Geometry: final body of the model. Coordinates: model frame, mm. A direction names the side the tool comes from. Coordinates: 2 decimals unless noted, no trailing zeros. Order: outer loops, then holes, each group sorted by start corner. A loop starts at its lowest first (then second) coordinate and runs counter-clockwise, first axis right, second up. Notation, with made-up numbers: (52, -25) - (111, -25) arc R13 ccw to (111, -4) - close; hole circle Ø8 at (15, 59.25). An arc over 180 degrees is marked (long way). Use a Markdown table: item, result. Add a question column.
```python
from build123d import *

# Parameters (mm, degrees)
SKETCH022_W            = 64
SKETCH022_H            = 64
PAD020_DEPTH           = 9
SKETCH023_R            = 1.6
POCKET003_DEPTH        = 9
SKETCH024_R            = 1.6
POCKET004_DEPTH        = 9
SKETCH025_R            = 3
POCKET005_DEPTH        = 5.5
SKETCH026_R            = 4.5
POCKET006_DEPTH        = 9
SKETCH030_R            = 1.55
POCKET009_DEPTH        = 9
SKETCH031_W            = 30
SKETCH031_H            = 27.227398
PAD022_DEPTH           = 9
SKETCH032_R            = 1.55
POCKET010_DEPTH        = 9
SKETCH066_W            = 16.8
SKETCH066_H            = 9
PAD040_DEPTH           = 8
PAD040_FACE8_W         = 9
PAD040_FACE8_H         = 16
PAD041_DEPTH           = 7
MIRRORED_FACE11_W      = 9
MIRRORED_FACE11_H      = 18
PAD042_DEPTH           = 7
PAD043_DEPTH           = 5.8
SKETCH068_R            = 2
POCKET027_DEPTH        = 5
LINEARPATTERN_COUNT    = 3
LINEARPATTERN_PITCH    = 6.4
SKETCH069_R            = 2
POCKET028_DEPTH        = 5
LINEARPATTERN001_COUNT = 3
LINEARPATTERN001_PITCH = 6.4
SKETCH071_W            = 10
SKETCH071_H            = 4
PAD044_DEPTH           = 5.8
SKETCH073_R            = 2
POCKET029_DEPTH        = 100
SKETCH074_W            = 11
SKETCH074_H            = 6
PAD045_DEPTH           = 50
SKETCH075_W            = 11
SKETCH075_H            = 2
POCKET030_DEPTH        = 12
SKETCH076_R            = 1.6
POCKET031_DEPTH        = 10
SKETCH083_R            = 3.25
POCKET035_DEPTH        = 4


with BuildPart() as part:
    # Sketch022 → Pad020 (new body)
    with BuildSketch(Plane.XZ):
        Rectangle(SKETCH022_W, SKETCH022_H)
    extrude(amount=PAD020_DEPTH)

    # Sketch023 (on Face5 of Pad020) → Pocket003 (cut)
    with BuildSketch(Plane(origin=(0, 0, 0), x_dir=(1, 0, 0), z_dir=(0, 1, 0))):
        with Locations((-9.5, 7.5)):
            Circle(SKETCH023_R)
        with Locations((-23.5, 7.5)):
            Circle(SKETCH023_R)
    extrude(amount=-POCKET003_DEPTH, mode=Mode.SUBTRACT)

    # Sketch024 (on Face4 of Pocket003) → Pocket004 (cut)
    with BuildSketch(Plane(origin=(0, 0, 0), x_dir=(1, 0, 0), z_dir=(0, 1, 0))):
        with Locations((1.4, 17.5)):
            Circle(SKETCH024_R)
        with Locations((18.9, -1.5)):
            Circle(SKETCH024_R)
    extrude(amount=-POCKET004_DEPTH, mode=Mode.SUBTRACT)

    # Sketch025 (on Face4 of Pocket004) → Pocket005 (cut)
    with BuildSketch(Plane(origin=(0, 0, 0), x_dir=(1, 0, 0), z_dir=(0, 1, 0))):
        with Locations((-23.5, 7.5)):
            Circle(SKETCH025_R)
        with Locations((-9.5, 7.5)):
            Circle(SKETCH025_R)
    extrude(amount=-POCKET005_DEPTH, mode=Mode.SUBTRACT)

    # Sketch026 (on Face4 of Pocket005) → Pocket006 (cut)
    with BuildSketch(Plane(origin=(0, 0, 0), x_dir=(1, 0, 0), z_dir=(0, 1, 0))):
        with Locations((0, -20)):
            Circle(SKETCH026_R)
        with Locations((20, 20)):
            Circle(SKETCH026_R)
        with Locations((-20, 20)):
            Circle(SKETCH026_R)
    extrude(amount=-POCKET006_DEPTH, mode=Mode.SUBTRACT)

    # Sketch030 (on Face5 of Pocket006) → Pocket009 (cut)
    with BuildSketch(Plane.XZ.offset(9)):
        with Locations((7.5, -7.5)):
            Circle(SKETCH030_R)
    extrude(amount=-POCKET009_DEPTH, mode=Mode.SUBTRACT)

    # Sketch031 (on Face5 of Pocket009) → Pad022 (join)
    with BuildSketch(Plane.XZ.offset(9)):
        with Locations((-1, 45.613699)):
            Rectangle(SKETCH031_W, SKETCH031_H)
    extrude(amount=-PAD022_DEPTH)

    # Sketch032 (on Face22 of Pad022) → Pocket010 (cut)
    with BuildSketch(Plane.XZ.offset(9)):
        with Locations((-9.5, 47.5)):
            Circle(SKETCH032_R)
        with Locations((7.5, 47.5)):
            Circle(SKETCH032_R)
    extrude(amount=-POCKET010_DEPTH, mode=Mode.SUBTRACT)

    # Sketch066 (on Face2 of Pocket010) → Pad040 (join)
    with BuildSketch(Plane(origin=(-32, 0, 0), x_dir=(0, 0, -1), z_dir=(-1, 0, 0))):
        with Locations((-30.6, 4.5)):
            Rectangle(SKETCH066_W, SKETCH066_H)
    pad040 = extrude(amount=PAD040_DEPTH)

    # Pad040 Face8 → Pad041 (add)
    with BuildSketch(Plane(origin=(-24, -4.5, 32), x_dir=(0, 1, 0), z_dir=(0, 0, 1))):
        Rectangle(PAD040_FACE8_W, PAD040_FACE8_H)
    extrude(amount=PAD041_DEPTH)

    # Mirrored: Pad040 across YZ
    add(pad040.mirror(Plane.YZ))

    # Mirrored Face11 → Pad042 (add)
    with BuildSketch(Plane(origin=(23, -4.5, 32), x_dir=(0, 1, 0), z_dir=(0, 0, 1))):
        Rectangle(MIRRORED_FACE11_W, MIRRORED_FACE11_H)
    extrude(amount=PAD042_DEPTH)

    # Sketch067 (on Face27 of Pad042) → Pad043 (join)
    with BuildSketch(Plane.XZ.offset(9)):
        Polygon((40, 39), (32, 39), (32, 22.2), (40, 22.2), (40, 24.2), (34, 24.2), (34, 37), (40, 37), align=None)
    pad043 = extrude(amount=PAD043_DEPTH)

    # Mirrored001: Pad043 across YZ
    add(pad043.mirror(Plane.YZ))

    # Sketch068 (on Face37 of Mirrored001) → Pocket027 (cut)
    with BuildSketch(Plane(origin=(-34, 0, 0), x_dir=(0, 0, -1), z_dir=(-1, 0, 0))):
        with Locations((-24.2, 11.9)):
            Circle(SKETCH068_R)
    pocket027 = extrude(amount=-POCKET027_DEPTH, mode=Mode.SUBTRACT)

    # LinearPattern: Pocket027 ×3
    with Locations(*[(0, 0, i * LINEARPATTERN_PITCH) for i in range(1, LINEARPATTERN_COUNT)]):
        add(pocket027, mode=Mode.SUBTRACT)

    # Sketch069 (on Face44 of LinearPattern) → Pocket028 (cut)
    with BuildSketch(Plane(origin=(34, 0, 0), x_dir=(0, 0, 1), z_dir=(1, 0, 0))):
        with Locations((37, 11.9)):
            Circle(SKETCH069_R)
    pocket028 = extrude(amount=-POCKET028_DEPTH, mode=Mode.SUBTRACT)

    # LinearPattern001: Pocket028 ×3
    with Locations(*[(0, 0, -i * LINEARPATTERN001_PITCH) for i in range(1, LINEARPATTERN001_COUNT)]):
        add(pocket028, mode=Mode.SUBTRACT)

    # Sketch071 (on Face35 of LinearPattern001) → Pad044 (join)
    with BuildSketch(Plane.XZ.offset(9)):
        with Locations((25, 21.7)):
            Rectangle(SKETCH071_W, SKETCH071_H)
        with Locations((25, -28.3)):
            Rectangle(SKETCH071_W, SKETCH071_H)
    pad044 = extrude(amount=PAD044_DEPTH)

    # Mirrored003: Pad044 across Sketch071 V_Axis
    add(pad044.mirror(Plane(origin=(0, -9, 0), x_dir=(0, -1, 0), z_dir=(1, 0, 0))))

    # Sketch073 (on Face49 of Mirrored003) → Pocket029 (cut)
    with BuildSketch(Plane(origin=(0, 0, 23.7), x_dir=(-1, 0, 0), z_dir=(0, 0, 1))):
        with Locations((-25, 11.9)):
            Circle(SKETCH073_R)
    pocket029 = extrude(amount=-POCKET029_DEPTH, mode=Mode.SUBTRACT)

    # Mirrored004: Pocket029 across YZ
    add(pocket029.mirror(Plane.YZ), mode=Mode.SUBTRACT)

    # Sketch074 (on Face15 of Mirrored004) → Pad045 (join)
    with BuildSketch(Plane(origin=(0, 0, -32), x_dir=(1, 0, 0), z_dir=(0, 0, -1))):
        with Locations((0, 3)):
            Rectangle(SKETCH074_W, SKETCH074_H)
    extrude(amount=PAD045_DEPTH)

    # Sketch075 (on Face41 of Pad045) → Pocket030 (cut)
    with BuildSketch(Plane(origin=(5.5, 0, 0), x_dir=(0, 0, 1), z_dir=(1, 0, 0))):
        with Locations((-74.5, 3)):
            Rectangle(SKETCH075_W, SKETCH075_H)
        with Locations((-45.5, 3)):
            Rectangle(SKETCH075_W, SKETCH075_H)
    extrude(amount=-POCKET030_DEPTH, mode=Mode.SUBTRACT)

    # Sketch076 (on Face30 of Pocket030) → Pocket031 (cut)
    with BuildSketch(Plane.XZ.offset(9)):
        with Locations((29, -12.3)):
            Circle(SKETCH076_R)
        with Locations((29, -20.3)):
            Circle(SKETCH076_R)
    extrude(amount=-POCKET031_DEPTH, mode=Mode.SUBTRACT)

    # Sketch083 (on Face32 of Pocket031) → Pocket035 (cut)
    with BuildSketch(Plane.XZ.offset(9)):
        with Locations((1.4, -17.5)):
            Circle(SKETCH083_R)
    extrude(amount=-POCKET035_DEPTH, mode=Mode.SUBTRACT)


solid = part.part
```
1) Line query: line 1 (X direction, y = -11.9, z = 21.95); line 2 (Z direction, x = 7.5, y = -7); line 3 (Y direction, x = -25, z = -27). Output: solid intervals per line, ascending. Write a range as from..to.
2) Draft query along Y for faces 1 (the flat face through (0, -4, -75)), 2 (the flat face through (-22, -5.5, -6)), 3 (the cylindrical face through (3.15, -7.03, -14.76)), 4 (the flat face through (25, -14.8, -28)). Return one class per face: released by +Y, released by -Y, zero draft, split by the parting line, or undercut.
3) Section query C-C (x = 1.4). Return the cut outline in (y, z).
4) First-contact query: pin 1 (7 mm diameter, centred on y = -6, z = 7, fed in from +X); pin 2 (7.5 mm diameter, centred on x = -23, y = -6, fed in from +Z); pin 3 (5.5 mm diameter, centred on x = 2, z = -46.5, fed in from -Y); pin 4 (5.5 mm diameter, centred on x = -2, z = -72.5, fed in from +Y). Flat tips, straight axial feed; report the tip coordinate or a pass-through.
5) Section query B-B (y = -7.5). Give the number of separate pieces and of enclosed holes in the cut face, and give its area (3 significant figures).
6) Section query A-A (z = -7.5). Return the cut outline in (x, y).
7) Access query for faces 5 (the flat face through (37, -12, 24.2)), 6 (the cylindrical face through (33.014, -9.948, 36.566)), 7 (the flat face through (3, -5, -19)), 8 (the flat face through (0, -2, -46)), 9 (the flat face through (-37, -12, 37)). Directions: +Z, -Z, +X, -X, +Y, -Y. A direction counts if a zero-diameter tool reaches every point of the face in a straight line with its end or side. Return the directions, or none.
8) Section query D-D (z = 30.6). Return the cut outline in (x, y).
From the geometry:
| question | item | result |
|---|---|---|
| 1 | line 1 | x = -30..-27, -23..-20, 20..23, 27..30 |
| 1 | line 2 | z = -32..-9.05, -5.95..45.95, 49.05..59.23 |
| 1 | line 3 | y = -14.8..-13.9, -9.9..0 |
| 2 | face 1 | undercut |
| 2 | face 2 | released by +Y |
| 2 | face 3 | zero draft |
| 2 | face 4 | released by -Y |
| 3 | outline | (-9, -32) - (-6, -32) - (-6, -82) - (0, -82) - (0, -19.1) - (-5, -19.1) - (-5, -20.75) - (-9, -20.75) - close; (-9, -14.25) - (-5, -14.25) - (-5, -15.9) - (0, -15.9) - (0, 15.72) - (-9, 15.72) - close; (-9, 24.28) - (0, 24.28) - (0, 59.23) - (-9, 59.23) - close; hole (-4, -80) - (-2, -80) - (-2, -69) - (-4, -69) - close; hole (-4, -51) - (-2, -51) - (-2, -40) - (-4, -40) - close |
| 4 | pin 1 | stops at x = 32 |
| 4 | pin 2 | stops at z = 39 |
| 4 | pin 3 | stops at y = -6 |
| 4 | pin 4 | stops at y = 0 |
| 5 | separate pieces | 1 |
| 5 | enclosed holes | 12 |
| 5 | area | 5,130 mm^2 |
| 6 | outline | (-32, -9) - (-25.1, -9) - (-25.1, -5.5) - (-26.5, -5.5) - (-26.5, 0) - (-32, 0) - close; (-21.9, -9) - (-11.1, -9) - (-11.1, -5.5) - (-12.5, -5.5) - (-12.5, 0) - (-20.5, 0) - (-20.5, -5.5) - (-21.9, -5.5) - close; (-7.9, -9) - (5.95, -9) - (5.95, 0) - (-6.5, 0) - (-6.5, -5.5) - (-7.9, -5.5) - close; (9.05, -9) - (32, -9) - (32, 0) - (9.05, 0) - close |
| 7 | face 5 | +X, -Y |
| 7 | face 6 | none |
| 7 | face 7 | -Y |
| 7 | face 8 | +X, -X |
| 7 | face 9 | -X, -Y |
| 8 | outline | (-40, -9) - (-34, -9) - (-34, -9.9) - (-32, -9.9) - (-32, -9) - (32, -9) - (32, -9.9) - (34, -9.9) - (34, -9) - (40, -9) - (40, 0) - (-40, 0) - close; (-34, -14.8) - (-32, -14.8) - (-32, -13.9) - (-34, -13.9) - close; (32, -14.8) - (34, -14.8) - (34, -13.9) - (32, -13.9) - close |
